```python
from build123d import *
from build123d.topology import SkipClean

# Parameters (mm, degrees)
SKETCH1_R           = 12.5
SKETCH1_R_2         = 5
BOSS_EXTRUDE1_DEPTH = 2
SKETCH3_R           = 12.665926605
SKETCH3_R_2         = 10.754079628
BOSS_EXTRUDE4_DEPTH = 1
REVOLVE1_ANGLE      = 5
CIRPATTERN1_COUNT   = 8
SKETCH5_R           = 1
BOSS_EXTRUDE5_DEPTH = 30
CIRPATTERN2_COUNT   = 6


with BuildPart() as part:
    # Sketch1 → Boss-Extrude1 (new body)
    with BuildSketch(Plane.XY):
        Circle(SKETCH1_R)
        Circle(SKETCH1_R_2, mode=Mode.SUBTRACT)
    extrude(amount=BOSS_EXTRUDE1_DEPTH)

    # Sketch3 → Boss-Extrude4 (add)
    with BuildSketch(Plane.XY.offset(2)):
        Circle(SKETCH3_R)
        Circle(SKETCH3_R_2, mode=Mode.SUBTRACT)
    extrude(amount=BOSS_EXTRUDE4_DEPTH)

    # Sketch4 → Revolve1 (revolve)
    with SkipClean():  # the faces are left unmerged after this step: merging them gives an invalid solid
        with BuildSketch(Plane(origin=(0, 0, 0), x_dir=(0, 0, -1), z_dir=(1, 0, 0))):
            Polygon((-9.330054786, 12.665926605), (-9.330054786, 10.565877972), (-2, 7.285294012), (-2, 12.665926605), align=None)
        revolve1 = revolve(axis=Axis((0, 0, 9.312529427), (0, 0, -1)), revolution_arc=REVOLVE1_ANGLE)
    add(part.part.scale(1), mode=Mode.REPLACE)  # the faces are merged on a copy

    # CirPattern1: Revolve1 ×8 about axis
    with SkipClean():  # the faces are left unmerged after this step: merging them gives an invalid solid
        cirpattern1_axis = Axis((0, 0, 0), (0, 0, 1))
        for i in range(1, CIRPATTERN1_COUNT):
            add(revolve1.rotate(cirpattern1_axis, i * 360 / CIRPATTERN1_COUNT))

    # Sketch5 → Boss-Extrude5 (add)
    with BuildSketch(Plane(origin=(0, 0, 0), x_dir=(-1, 0, 0), z_dir=(0, 0, -1))):
        with Locations(Location((0, 8.75, 0), (0, 0, 180))):
            Circle(SKETCH5_R)
    boss_extrude5 = extrude(amount=BOSS_EXTRUDE5_DEPTH)

    # CirPattern2: Boss-Extrude5 ×6 about axis
    cirpattern2_axis = Axis((0, 0, 0), (0, 0, 1))
    for i in range(1, CIRPATTERN2_COUNT):
        add(boss_extrude5.rotate(cirpattern2_axis, i * 360 / CIRPATTERN2_COUNT))

    # Mirror4: part across plane


with BuildPart() as part_1:
    add(part.part)
    add(part.part.mirror(Plane.XY.offset(-30)))


solid = part_1.part
```
Here's how the part is built. I have some questions about the finished solid (model axes, mm). A direction names the side the tool comes from. Coordinates: 2 decimals unless noted, no trailing zeros. Order: outer loops, then holes, each group sorted by start corner. A loop starts at its lowest first (then second) coordinate and runs counter-clockwise, first axis right, second up.
1) Which directions (+Z, -Z, +X, -X, +Y, -Y) give clear straight access to the entire face, cutting with the end or side of a thin tool? Please do faces 4 (the face through (-3.629, 10.123, -62.493)), 5 (the face through (4, -11, 3)), 6 (the face through (-10.123, -3.629, 2.493)), 7 (the face through (-4, 11, -63)).
2) I need wall thicknesses on line 1 (Z direction, x = -10.5, y = -5.75); line 2 (Z direction, x = 3.5, y = -7.75); line 3 (Y direction, x = 0, z = -61.1). Which ranges of each line are inside material? Lowest first, please.
3) Will these pins go through, and if not, where does the flat tip stop? pin 1 (3 mm diameter, centred on x = 1.5, y = -6.5, fed in from +Z); pin 2 (10 mm diameter, centred on y = 0.5, z = -22.5, fed in from +X); pin 3 (5 mm diameter, centred on x = 10.5, y = 5, fed in from +Z).
4) Imagine slicing it at A-A on z = -54. List the corners of the cut face in (x, y) for me (3 decimals).
5) We'd pull the mould along X, two halves only. Please class faces 1 (the face through (5, -2, 2)), 2 (the face through (-10, 5, -63)), 3 (the face through (-1.08, -4.88, -60.99)): +X half, -X half, draft (parallel to the pull), parting line (faces both ways), or undercut.
Response values:
1. face 4: -Z
1. face 5: +Z, -Y
1. face 6: +Z
1. face 7: -Z, +Y
2. line 1: z = -63 to -60, 0 to 3
2. line 2: z = -62 to -60, 0 to 2
2. line 3: y = -12.5 to -5, 5 to 12.5
3. pin 1: stops at z = 2
3. pin 2: stops at x = 8.58
3. pin 3: stops at z = 3
4. outline: circle Ø2 at (-7.578, -4.375); circle Ø2 at (-7.578, 4.375); circle Ø2 at (0, -8.75); circle Ø2 at (0, 8.75); circle Ø2 at (7.578, -4.375); circle Ø2 at (7.578, 4.375)
5. face 1: undercut
5. face 2: draft
5. face 3: undercut
